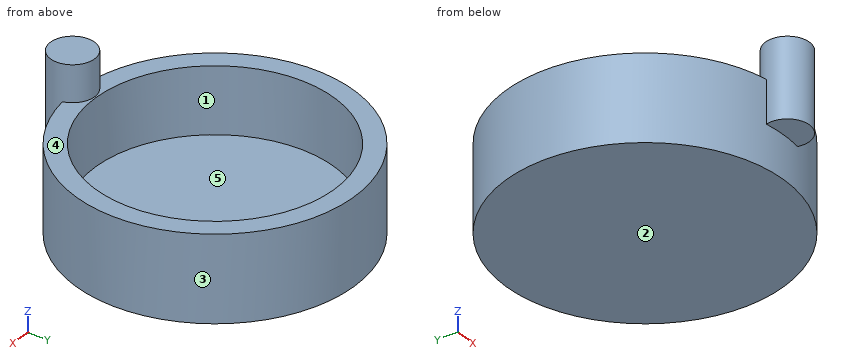
```python
from build123d import *

# Parameters (mm, degrees)
F0_R     = 10.6
F1_DEPTH = 3.25
F2_T     = -1.5
F3_R     = 1.676803
F4_DEPTH = 6


with BuildPart() as f1:
    # F0 (on Top) → F1 (new body, symmetric)
    with BuildSketch(Plane.XY):
        Circle(F0_R)
    extrude(amount=F1_DEPTH, both=True)

    # F2
    f2_openings = [f1.faces().sort_by_distance(p)[0] for p in [
        (0, 0, 3.25),
    ]]
    offset(amount=F2_T, openings=f2_openings)

    # F3 (on Top) → F4 (join)
    with BuildSketch(Plane.XY):
        with Locations((0, -10.890958)):
            Circle(F3_R)
    extrude(amount=F4_DEPTH)


solid = f1.part
```
Part model, mm, in its own coordinate system. Face numbers are marked on the shaded views. A direction names the side the tool comes from. Round coordinates to 2 decimals unless told otherwise and drop trailing zeros. Loops run counter-clockwise (first coordinate to the right, second up) from the corner with the lowest first, then second, coordinate; pieces in that order, holes last. Notation, with made-up numbers: (61.25, 77) -> (67.25, 77) arc R29 cw to (67.25, 105) -> close; hole circle Ø11 at (-39.5, 67). An arc over 180 degrees is marked (long way). Use one line per item in the form item = value. Start each with the question number.
Item 1: Drill centre lines: line 1 along Y through (x, z) = (0, 0.6); line 2 along Y through (x, z) = (0, -0.6); line 3 along X through (y, z) = (-6, 1). Where is each one in solid material? Low to high.
Item 2: Drop flat-ended pins along their axis: pin 1 Ø2 at (x, y) = (-2.5, -2) entering from +Z; pin 2 Ø6.5 at (x, y) = (5, 5) entering from +Z; pin 3 Ø1.7 at (x, y) = (0.5, -11.5) entering from -Z. Give the stop position or say it passes through.
Item 3: Band-saw the part on C-C (z = -0.75). List the corners of the cut face in (x, y).
Item 4: Band-saw the part on D-D (x = 6.75). List the corners of the cut face in (y, z).
Item 5: Two-plate mould, pull along X, no slides. Class the marked faces 3, 4 and 5: released by +X, released by -X, zero draft, split by the parting line, or undercut.
Item 6: Band-saw the part on B-B (x = 0). List the corners of the cut face in (y, z).
Item 7: Band-saw the part on A-A (y = 0). List the corners of the cut face in (x, z).
Item 8: Tool access for the marked faces 1 and 2: list every direction of +Z, -Z, +X, -X, +Y, -Y with a clear straight run to the whole face (end or side of a thin tool).
Data:
q1.line_1 = -12.57 to -9.1, 9.1 to 10.6
q1.line_2 = -10.6 to -9.1, 9.1 to 10.6
q1.line_3 = -8.74 to -6.84, 6.84 to 8.74
q2.pin_1 = -1.75
q2.pin_2 = 3.25
q2.pin_3 = 0
q3.outline = circle Ø21.2 at (0, 0); hole circle Ø18.2 at (0, 0)
q4.outline = (-8.17, -3.25) -> (8.17, -3.25) -> (8.17, 3.25) -> (6.1, 3.25) -> (6.1, -1.75) -> (-6.1, -1.75) -> (-6.1, 3.25) -> (-8.17, 3.25) -> close
q5.face_3 = split by the parting line
q5.face_4 = zero draft
q5.face_5 = undercut
q6.outline = (-12.57, 0) -> (-10.6, 0) -> (-10.6, -3.25) -> (10.6, -3.25) -> (10.6, 3.25) -> (9.1, 3.25) -> (9.1, -1.75) -> (-9.1, -1.75) -> (-9.1, 3.25) -> (-9.21, 3.25) -> (-9.21, 6) -> (-12.57, 6) -> close
q7.outline = (-10.6, -3.25) -> (10.6, -3.25) -> (10.6, 3.25) -> (9.1, 3.25) -> (9.1, -1.75) -> (-9.1, -1.75) -> (-9.1, 3.25) -> (-10.6, 3.25) -> close
q8.face_1 = +Z
q8.face_2 = -Z, +X, -X, +Y, -Y
